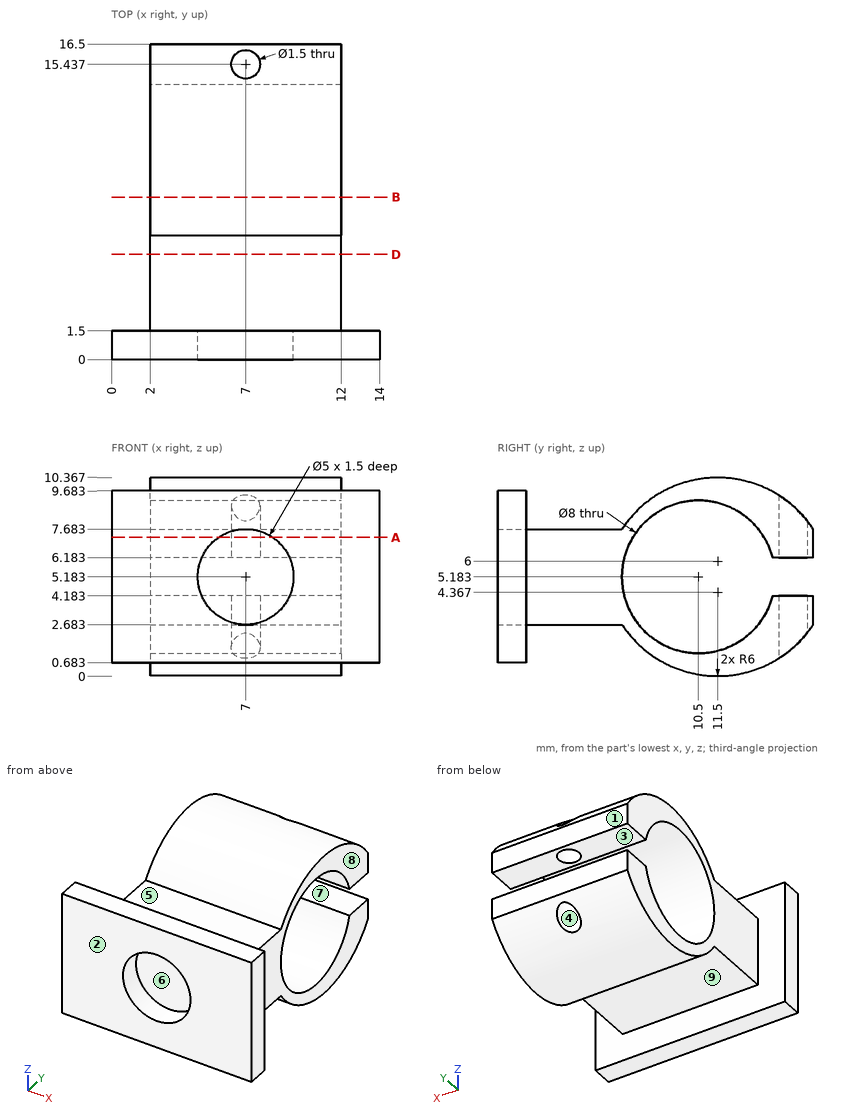
Check sheet for the drawn part. Datum: minimum x, y, z corner. Units: mm. A direction names the side the tool comes from. Round coordinates to 2 decimals unless told otherwise and drop trailing zeros. Loops run counter-clockwise (first coordinate to the right, second up) from the corner with the lowest first, then second, coordinate; pieces in that order, holes last.
Item 1: Cross-section at D-D on y = 5.5. Record the boundary of the cut face in (x, z), then the cut area to 3 significant figures.
Item 2: Access from +Z, -Z, +X, -X, +Y, -Y to the whole of each face (thin tool, end or side, straight path). Record for the marked faces 5, 6, 7, 8 and 9.
Item 3: Mould release check, pull along Y, two halves, no side actions. Record for the marked faces 1, 2, 3 and 4: pulls with the +Y half, pulls with the -Y half, needs draft (parallel to the pull), parting line crosses it, or undercut.
Item 4: Gauge pin test, flat ends, axial feed: pin 1 (2.5 mm diameter, centred on x = 5.5, y = 16, fed in from -Z) (1 decimal); pin 2 (2 mm diameter, centred on y = 11, z = 1, fed in from +X); pin 3 (5.5 mm diameter, centred on x = 8.5, y = 4.5, fed in from -Z) (1 decimal). Record the tip position at first contact, or that the pin passes through.
Item 5: Cross-section at A-A on z = 7.25. Count the separate pieces of the cut face and the enclosed holes in it.
Item 6: Cross-section at B-B on y = 8.5. Record the boundary of the cut face in (x, z).
Item 7: Thickness scan on line 1 (Z direction, x = 7, y = 0.8); line 2 (Y direction, x = 6.5, z = 8.75) (1 decimal); line 3 (X direction, y = 15.5, z = 3). Record the ranges inside material, lowest first.
Answer sheet:
1. outline: (2, 2.68) - (12, 2.68) - (12, 7.68) - (2, 7.68) - close
1. area: 50.0 mm2
2. face 5: +Z, +X, -X
2. face 6: -Y
2. face 7: +X, -X, +Y
2. face 8: +Z, -Z, +X, +Y
2. face 9: -Z, +X, -X
3. face 1: pulls with the +Y half
3. face 2: pulls with the -Y half
3. face 3: needs draft
3. face 4: undercut
4. pin 1: stops at z = 1
4. pin 2: stops at x = 12
4. pin 3: stops at z = 1.8
5. separate pieces: 2
5. enclosed holes: 1
6. outline: (2, 0.8) - (12, 0.8) - (12, 1.72) - (2, 1.72) - close; (2, 8.65) - (12, 8.65) - (12, 9.56) - (2, 9.56) - close
7. line 1: z = 0.68 to 2.68, 7.68 to 9.68
7. line 2: y = 0 to 1.5, 7.4 to 8.7, 12.3 to 14.9
7. line 3: x = 2 to 6.25, 7.75 to 12
